The drawing under review shows one solid part. Ordinate dimensions are in mm from its lowest x, y, z. Give positions to 0.01 mm unless a question says otherwise; leave off trailing zeros. Loops run counter-clockwise (first coordinate to the right, second up) from the corner with the lowest first, then second, coordinate; pieces in that order, holes last. Notation, with made-up numbers: (48.5, 6) - (66.5, 6) arc R20 ccw to (66.5, 41) - close; hole circle Ø11 at (63.25, 88.5). An arc over 180 degrees is marked (long way). Put each result on its own line as item: value. Start each with the question number.
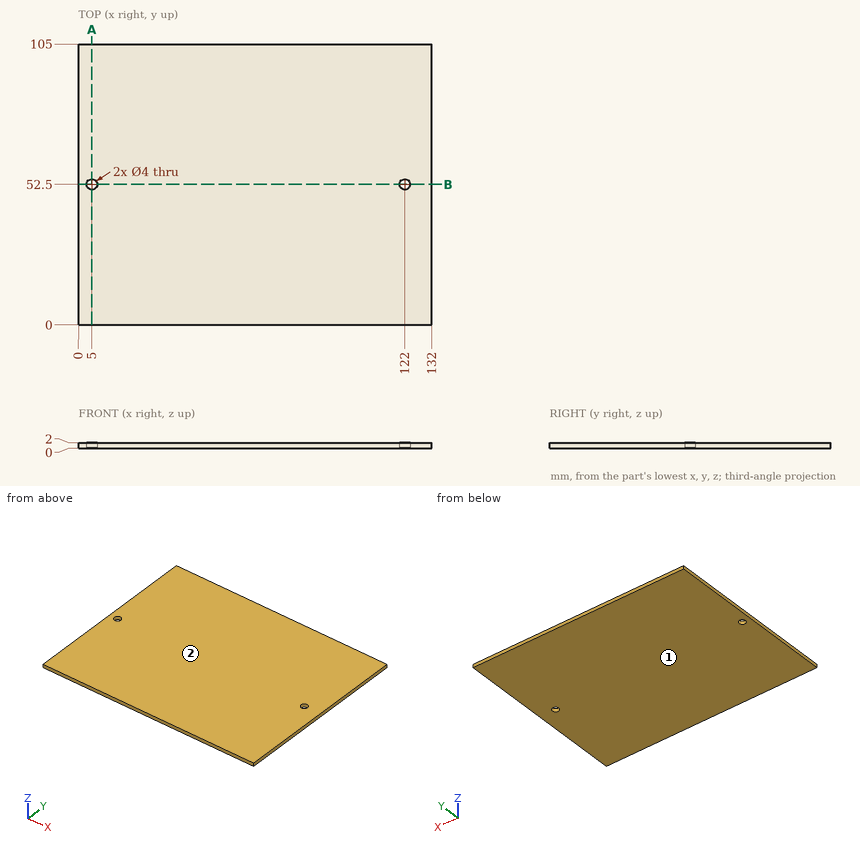
Item 1: Consider section A-A (x = 5). State the section outline as (y, z) points, plus the area to 3 significant figures.
Item 2: For L1, parallel to Y at x = 5, z = 1.25; L2, parallel to X at y = 52, z = 1.4, list the stretches that pass through material, from the lowest coordinate up. Write a range as from..to.
Item 3: Consider section B-B (y = 52.5). State the section outline as (x, z) points.
Item 4: Mouldability with a two-part tool opening along Z and no side actions: class the marked faces 1 and 2 as pulls with the +Z half, pulls with the -Z half, needs draft (parallel to the pull), parting line crosses it, or undercut.
Geometry says:
1. outline: (0, 0) - (50.5, 0) - (50.5, 2) - (0, 2) - close; (54.5, 0) - (105, 0) - (105, 2) - (54.5, 2) - close
1. area: 202 mm2
2. L1: y = 0..50.5, 54.5..105
2. L2: x = 0..3.06, 6.94..120.06, 123.94..132
3. outline: (0, 0) - (3, 0) - (3, 2) - (0, 2) - close; (7, 0) - (120, 0) - (120, 2) - (7, 2) - close; (124, 0) - (132, 0) - (132, 2) - (124, 2) - close
4. face 1: pulls with the -Z half
4. face 2: pulls with the +Z half
